Work out the finished part from the listing and answer in its coordinate system (mm). A direction names the side the tool comes from. Round coordinates to 2 decimals unless told otherwise and drop trailing zeros. Order: outer loops, then holes, each group sorted by start corner. A loop starts at its lowest first (then second) coordinate and runs counter-clockwise, first axis right, second up. Notation, with made-up numbers: M 23,-28 L 59,-28 A15 ccw 59,1 Z; hole C -31,-15.5 d9. An arc over 180 degrees is marked long. Answer as a JSON object with one key per item and string values. Group by question number.
from build123d import *

# Parameters (mm, degrees)
BOSS_EXTRUDE1_DEPTH = 15.85
SKETCH2_R           = 2.45
SKETCH2_R_2         = 1.46
BOSS_EXTRUDE2_DEPTH = 1.8
SKETCH3_R           = 2.45
BOSS_EXTRUDE3_DEPTH = 1.8
SHELL1_START        = -3.15
SHELL1_OUTLINE_W    = 12.85
SHELL1_OUTLINE_H    = 6.65
SHELL1_DEPTH        = 1.65
SHELL1_START_2      = -1.5
SHELL1_2_OUTLINE_R  = 0.95
SHELL1_2_DEPTH      = 1.8


# Read off the part's stored shape, not the designer's step: Shell1
with BuildPart() as part:
    # Sketch1 → Boss-Extrude1 (new body)
    with BuildSketch(Plane(origin=(0, 0, 0), x_dir=(0, 0, -1), z_dir=(1, 0, 0))):
        Polygon((0, 0), (0, -9.65), (3.15, -9.65), (3.15, -1.6), (7.8, -1.6), (7.8, 0), align=None)
    extrude(amount=-BOSS_EXTRUDE1_DEPTH)

    # Sketch2 → Boss-Extrude2 (add)
    # profile 1 of 2: a face of its own
    with BuildSketch(Plane(origin=(0, 0, 0), x_dir=(1, 0, 0), z_dir=(0, 1, 0))):
        with Locations(Location((-11.8875, 3.9, 0), (0, 0, 270))):
            Circle(SKETCH2_R)
        with Locations(Location((-11.8875, 3.9, 0), (0, 0, 270))):
            Circle(SKETCH2_R_2, mode=Mode.SUBTRACT)
    # profile 2 of 2: a face of its own
    with BuildSketch(Plane(origin=(0, 0, 0), x_dir=(1, 0, 0), z_dir=(0, 1, 0))):
        with Locations(Location((-3.9625, 3.9, 0), (0, 0, 270))):
            Circle(SKETCH2_R)
        with Locations(Location((-3.9625, 3.9, 0), (0, 0, 270))):
            Circle(SKETCH2_R_2, mode=Mode.SUBTRACT)
    extrude(amount=BOSS_EXTRUDE2_DEPTH)

    # Sketch3 → Boss-Extrude3 (add)
    with BuildSketch(Plane.XY):
        with Locations((-11.8875, -5.625)):
            Circle(SKETCH3_R)
        with Locations((-3.9625, -5.625)):
            Circle(SKETCH3_R)
    extrude(amount=BOSS_EXTRUDE3_DEPTH)

    # Shell1 outline → Shell1 (cut)
    with BuildSketch(Plane.XY.offset(SHELL1_START)):
        with Locations((-7.925, -4.825)):
            Rectangle(SHELL1_OUTLINE_W, SHELL1_OUTLINE_H)
    extrude(amount=SHELL1_DEPTH, mode=Mode.SUBTRACT)

    # Shell1 2 outline → Shell1 2 (cut)
    with BuildSketch(Plane.XY.offset(SHELL1_START_2)):
        with Locations((-11.8875, -5.625)):
            Circle(SHELL1_2_OUTLINE_R)
        with Locations((-3.9625, -5.625)):
            Circle(SHELL1_2_OUTLINE_R)
    extrude(amount=SHELL1_2_DEPTH, mode=Mode.SUBTRACT)


solid = part.part
Item 1: Find section D-D (y = -7.25). Give the vertices of the cut face in (x, z), and give its area (3 significant figures).
Item 2: Find section B-B (x = -9.25). Give the vertices of the cut face in (y, z), and give its area (3 significant figures).
Item 3: A tool of negligible diameter and unlimited length cuts with its end or side. For faces 5 (the flat face through (-8, -1.6, -5)), 6 (the flat face through (-8, -8.15, -2)), 7 (the flat face through (-8, 0, -4)), from which of +Z, -Z, +X, -X, +Y, -Y can it reach the whole face along a straight path? Write none if from no direction.
Item 4: Find section C-C (z = -2.75). Give the vertices of the cut face in (x, y), and give its area (3 significant figures).
Item 5: Consider L1, parallel to X at y = 0.9, z = -3.9; L2, parallel to Y at x = -5.25, z = -2; L3, parallel to X at y = -5.25, z = -0.25. Determine where each line is inside the solid, lowest interval first.
Item 6: Each of these flat-tipped pins is pushed along its axis until it touches: pin 1 (4 mm diameter, centred on x = -12, z = -4.5, fed in from -Y); pin 2 (1.7 mm diameter, centred on x = -3.96, y = -5.62, fed in from -Z); pin 3 (3.5 mm diameter, centred on x = -6.5, y = -4, fed in from -Z). Where does it stop, or does it pass through?
Item 7: The mould has two halves that part along Z. Classify faces 1 (the cylindrical face through (-5.77, -3.97, 0.89)), 2 (the cylindrical face through (-13.378, 0.887, -5.844)), 3 (the flat face through (-8, -1.5, -2)), 4 (the flat face through (-8, -5, 0)): +Z half, -Z half, draft (parallel to the pull), parting line (faces both ways), or undercut.
Item 8: Find section A-A (z = -3.9). Give the vertices of the cut face in (x, y).
Responses:
{
 "1": {"outline": "M -15.85,-3.15 L -14.35,-3.15 L -14.35,-1.5 L -1.5,-1.5 L -1.5,-3.15 L 0,-3.15 L 0,0 L -2.13,0 L -2.13,1.8 L -5.8,1.8 L -5.8,0 L -10.05,0 L -10.05,1.8 L -13.72,1.8 L -13.72,0 L -15.85,0 Z", "area": "41.9 mm^2"},
 "2": {"outline": "M -9.65,-3.15 L -8.15,-3.15 L -8.15,-1.5 L -1.5,-1.5 L -1.5,-3.15 L -1.6,-3.15 L -1.6,-7.8 L 0,-7.8 L 0,0 L -9.65,0 Z", "area": "26.9 mm^2"},
 "3": {"face 5": "-Z, +X, -X, -Y", "face 6": "-Z", "face 7": "+Y"},
 "4": {"outline": "M -15.85,-9.65 L 0,-9.65 L 0,0 L -1.8,0 L -1.8,1.8 L -3.06,1.8 L -3.06,0 L -4.86,0 L -4.86,1.8 L -6.13,1.8 L -6.13,0 L -9.72,0 L -9.72,1.8 L -10.99,1.8 L -10.99,0 L -12.79,0 L -12.79,1.8 L -14.05,1.8 L -14.05,0 L -15.85,0 Z; hole M -14.35,-8.15 L -1.5,-8.15 L -1.5,-1.5 L -14.35,-1.5 Z", "area": "76.6 mm^2"},
 "5": {"L1": "x = -14.34 to -13.35, -10.43 to -9.44, -6.41 to -5.42, -2.5 to -1.51", "L2": "y = -9.65 to -8.15, -1.5 to 1.8", "L3": "x = -15.85 to -12.76, -11.01 to -4.84, -3.09 to 0"},
 "6": {"pin 1": "stops at y = -9.65", "pin 2": "stops at z = 0.3", "pin 3": "stops at z = -1.5"},
 "7": {"face 1": "draft", "face 2": "parting line", "face 3": "undercut", "face 4": "+Z half"},
 "8": {"outline": "M -15.85,-1.6 L 0,-1.6 L 0,0 L -1.51,0 L -1.51,1.8 L -2.5,1.8 L -2.5,0 L -5.42,0 L -5.42,1.8 L -6.41,1.8 L -6.41,0 L -9.44,0 L -9.44,1.8 L -10.43,1.8 L -10.43,0 L -13.35,0 L -13.35,1.8 L -14.34,1.8 L -14.34,0 L -15.85,0 Z"}
}
